```python
from build123d import *

# Parameters (mm, degrees)
F1_DEPTH  = 50
F3_R      = 3.5
F4_DEPTH  = 25
F5_START  = 14
F5_DEPTH  = 18
F7_W      = 3.5
F7_H      = 6
F8_DEPTH  = 12.5
F10_W     = 3.5
F10_H     = 6
F11_DEPTH = 12.5


with BuildPart() as f1:
    # F0 (on Top) → F1 (new body)
    with BuildSketch(Plane.XY):
        with BuildLine():
            ThreePointArc((-25, -7.5), (0, -3.3285658241), (25, -7.5))
            Line((25, -7.5), (25, 7.5))
            Line((25, 7.5), (-25, 7.5))
            Line((-25, 7.5), (-25, -7.5))
        make_face()
    extrude(amount=F1_DEPTH)

    # F3 (on face) → F4 (cut)
    with BuildSketch(Plane(origin=(0, 5.625, -3.2475952642), x_dir=(1, 0, 0), z_dir=(0, -0.8660254038, 0.5))):
        with Locations((0, 20)):
            Circle(F3_R)
    extrude(amount=F4_DEPTH, mode=Mode.SUBTRACT)

    # F3 (on face) → F5 (cut)
    with BuildSketch(Plane(origin=(0, 5.625, -3.2475952642), x_dir=(1, 0, 0), z_dir=(0, -0.8660254038, 0.5)).offset(F5_START)):
        Polygon((-5.75, 23.3197640478), (-5.75, 16.6802359522), (0, 13.3604719043), (5.75, 16.6802359522), (5.75, 23.3197640478), (0, 26.6395280957), align=None)
        with Locations((0, 20)):
            Circle(F3_R, mode=Mode.SUBTRACT)
        with Locations((0, 20)):
            Circle(F3_R)
    extrude(amount=F5_DEPTH, mode=Mode.SUBTRACT)

    # F7 (on face) → F8 (cut, symmetric)
    with BuildSketch(Plane(origin=(8.75, -8.75, 0), x_dir=(-0.7071067812, -0.7071067812, 0), z_dir=(-0.7071067812, 0.7071067812, 0))):
        with Locations((-18, 10)):
            Rectangle(F7_W, F7_H)
        with Locations((-18, 40)):
            Rectangle(F7_W, F7_H)
    extrude(amount=F8_DEPTH, both=True, mode=Mode.SUBTRACT)

    # F10 (on face) → F11 (cut, symmetric)
    with BuildSketch(Plane(origin=(-8.75, -8.75, 0), x_dir=(0.7071067812, -0.7071067812, 0), z_dir=(-0.7071067812, -0.7071067812, 0))):
        with Locations((-18, 10)):
            Rectangle(F10_W, F10_H)
        with Locations((-18, 40)):
            Rectangle(F10_W, F10_H)
    extrude(amount=F11_DEPTH, both=True, mode=Mode.SUBTRACT)


solid = f1.part
```
Build history of the part. All positions in model axes, mm. A direction names the side the tool comes from. Coordinates: 2 decimals unless noted, no trailing zeros. Order: outer loops, then holes, each group sorted by start corner. A loop starts at its lowest first (then second) coordinate and runs counter-clockwise, first axis right, second up.
Item 1: Mould opens along X. For faces 4 (the flat face through (-25, 0, 25)), 5 (the flat face through (0, 7.5, 25)), 6 (the flat face through (21, 4, 13)) say: released by +X, released by -X, zero draft, split by the parting line, or undercut.
Filled in:
face 4: released by -X
face 5: zero draft
face 6: undercut
Item 2: Saw through at C-C on y = -1.25. List the corners of the cut face in (x, z).
Filled in:
outline: (-25, 0) - (25, 0) - (25, 7) - (24.23, 7) - (24.23, 13) - (25, 13) - (25, 37) - (24.23, 37) - (24.23, 43) - (25, 43) - (25, 50) - (-25, 50) - (-25, 43) - (-24.23, 43) - (-24.23, 37) - (-25, 37) - (-25, 13) - (-24.23, 13) - (-24.23, 7) - (-25, 7) - close; hole (-5.75, 19.98) - (0, 16.15) - (5.75, 19.98) - (5.75, 27.65) - (0, 31.48) - (-5.75, 27.65) - close
Item 3: Saw through at B-B on x = 2.5. List the corners of the cut face in (y, z).
Filled in:
outline: (-3.37, 0) - (7.5, 0) - (7.5, 15.94) - (2.28, 18.95) - (0.9, 16.57) - (-3.37, 19.04) - close; (-3.37, 31.04) - (6.1, 25.57) - (4.73, 23.19) - (7.5, 21.59) - (7.5, 50) - (-3.37, 50) - close
Item 4: Saw through at A-A on z = 8.5. List the corners of the cut face in (x, y).
Filled in:
outline: (-25, -7.5) arc R77 cw to (25, -7.5) - (25, -2.02) - (15.48, 7.5) - (-15.48, 7.5) - (-25, -2.02) - close; (-25, 2.93) - (-20.43, 7.5) - (-25, 7.5) - close; (20.43, 7.5) - (25, 2.93) - (25, 7.5) - close
Item 5: Drill centre lines: L1, parallel to Z at x = 22.5, y = 4; L2, parallel to X at y = 6.25, z = 42.5; L3, parallel to Y at x = 0.5, z = 33.5. Where is each one in solid material? Low to high.
Filled in:
L1: z = 0 to 7, 13 to 37, 43 to 50
L2: x = -25 to -21.68, -16.73 to 16.73, 21.68 to 25
L3: y = -3.33 to 7.5
Item 6: Tool access for faces 1 (the flat face through (-2.92, -1.03, 17.97)), 2 (the flat face through (-2.835, 0.999, 28.294)), 3 (the flat face through (0, 2, 0)): list every direction of +Z, -Z, +X, -X, +Y, -Y with a clear straight run to the whole face (end or side of a thin tool).
Filled in:
face 1: none
face 2: -Y
face 3: -Z, +X, -X, +Y, -Y
Item 7: Drop a flat-ended pin along its axis: pin 1 Ø2 at (x, z) = (-7, 10.5) entering from -Y. Give the stop position or say it passes through.
Filled in:
pin 1: stops at y = -3.75
Item 8: Saw through at D-D on z = 25. List the corners of the cut face in (x, y).
Filled in:
outline: (-25, -7.5) arc R77 cw to (-5.75, -3.54) - (-5.75, 3.34) - (-3.65, 5.77) - (3.65, 5.77) - (5.75, 3.34) - (5.75, -3.54) arc R77 cw to (25, -7.5) - (25, 7.5) - (-25, 7.5) - close
